from build123d import *

# Parameters (mm, degrees)
F1_DEPTH = 12
F2_DEPTH = 2.5
F3_DEPTH = 1.5


# Not quite as in the source:
# - a feature names something its author has since deleted; it is built from what else it names


with BuildPart() as f1:
    # F0 (on Top) → F1 (new body)
    with BuildSketch(Plane.XY):
        with BuildLine():
            Line((-1.9364916731, 0.5), (1.9364916731, 0.5))
            ThreePointArc((1.9364916731, 0.5), (0, 2), (-1.9364916731, 0.5))
        make_face()
        with BuildLine():
            ThreePointArc((2, 0), (1.9840593925, 0.252008585), (1.9364916731, 0.5))
            Line((1.9364916731, 0.5), (-1.9364916731, 0.5))
            ThreePointArc((-1.9364916731, 0.5), (-2, 0), (-1.9364916731, -0.5))
            Line((-1.9364916731, -0.5), (1.9364916731, -0.5))
            ThreePointArc((1.9364916731, -0.5), (1.9840593925, -0.252008585), (2, 0))
        make_face()
        with BuildLine():
            ThreePointArc((-1.9364916731, -0.5), (0, -2), (1.9364916731, -0.5))
            Line((1.9364916731, -0.5), (-1.9364916731, -0.5))
        make_face()
    extrude(amount=-F1_DEPTH)

    # F0 (on Top) → F2 (join)
    with BuildSketch(Plane.XY):
        with BuildLine():
            ThreePointArc((-3.9686269666, -0.5), (0, -4), (3.9686269666, -0.5))
            Line((3.9686269666, -0.5), (1.9364916731, -0.5))
            ThreePointArc((1.9364916731, -0.5), (0, -2), (-1.9364916731, -0.5))
            Line((-1.9364916731, -0.5), (-3.9686269666, -0.5))
        make_face()
        with BuildLine():
            Line((1.9364916731, 0.5), (3.9686269666, 0.5))
            ThreePointArc((3.9686269666, 0.5), (0, 4), (-3.9686269666, 0.5))
            Line((-3.9686269666, 0.5), (-1.9364916731, 0.5))
            ThreePointArc((-1.9364916731, 0.5), (0, 2), (1.9364916731, 0.5))
        make_face()
        with BuildLine():
            Line((-1.9364916731, 0.5), (1.9364916731, 0.5))
            ThreePointArc((1.9364916731, 0.5), (0, 2), (-1.9364916731, 0.5))
        make_face()
        with BuildLine():
            ThreePointArc((-1.9364916731, -0.5), (0, -2), (1.9364916731, -0.5))
            Line((1.9364916731, -0.5), (-1.9364916731, -0.5))
        make_face()
    extrude(amount=F2_DEPTH)

    # F0 (on Top) → F3 (join)
    with BuildSketch(Plane.XY):
        with BuildLine():
            Line((-1.9364916731, 0.5), (-3.9686269666, 0.5))
            ThreePointArc((-3.9686269666, 0.5), (-4, 0), (-3.9686269666, -0.5))
            Line((-3.9686269666, -0.5), (-1.9364916731, -0.5))
            ThreePointArc((-1.9364916731, -0.5), (-2, 0), (-1.9364916731, 0.5))
        make_face()
        with BuildLine():
            ThreePointArc((2, 0), (1.9840593925, 0.252008585), (1.9364916731, 0.5))
            Line((1.9364916731, 0.5), (-1.9364916731, 0.5))
            ThreePointArc((-1.9364916731, 0.5), (-2, 0), (-1.9364916731, -0.5))
            Line((-1.9364916731, -0.5), (1.9364916731, -0.5))
            ThreePointArc((1.9364916731, -0.5), (1.9840593925, -0.252008585), (2, 0))
        make_face()
        with BuildLine():
            ThreePointArc((3.9686269666, -0.5), (3.9921490369, -0.2504916502), (4, 0))
            ThreePointArc((4, 0), (3.9921490369, 0.2504916502), (3.9686269666, 0.5))
            Line((3.9686269666, 0.5), (1.9364916731, 0.5))
            ThreePointArc((1.9364916731, 0.5), (1.9840593925, 0.252008585), (2, 0))
            ThreePointArc((2, 0), (1.9840593925, -0.252008585), (1.9364916731, -0.5))
            Line((1.9364916731, -0.5), (3.9686269666, -0.5))
        make_face()
    extrude(amount=F3_DEPTH)


solid = f1.part
Model file for the job. Use its own axes, mm. A direction names the side the tool comes from. Coordinates: 2 decimals unless noted, no trailing zeros. Write each loop counter-clockwise with the first axis right and the second up, starting at its lowest first coordinate (ties: lowest second). Pieces come first, ordered by that corner, then holes. Notation, with made-up numbers: (-6, 26.25) - (16, 26.25) arc R31 ccw to (16, 55.25) - close; hole circle Ø4 at (62, 67). An arc over 180 degrees is marked (long way). Write each question's results on one line, items separated by ' | '. Start each with the question number.
1) Cut at B-B (z = 1). Write the cut outline in (x, y), then the cut area to 3 significant figures.
2) Probe line 1 along X through (y, z) = (-0.5, -2.25); line 2 along Z through (x, y) = (1, 3.75). List the from-to ranges inside material, lowest first. Write a range as from..to.
3) Cut at D-D (z = -10.5). Write the cut outline in (x, y).
4) Mould opens along Y. For faces 4 (the face through (0, 0.5, 2)), 5 (the face through (0, 2, 2.5)) say: pulls with the +Y half, pulls with the -Y half, needs draft (parallel to the pull), parting line crosses it, or undercut.
5) Cut at C-C (y = -1.25). Write the cut outline in (x, z), then the cut area to 3 significant figures.
6) Flat gauge pins, fed straight in: P1, Ø0.5, axis at x = 0.5, y = 0, coming from the +Z side; P2, Ø0.8, axis at x = 1, z = 2, coming from the -Y side; P3, Ø3, axis at y = -1, z = -7, coming from the +X side. Where does each tip first touch, or does it go through?
7) 3-axis set-ups, long thin cutter, end or side, ignore diameter. For faces 1 (the face through (0, -2, 2.5)), 2 (the face through (1, 2, 0)), 3 (the face through (0, -0.5, 2)): which of +Z, -Z, +X, -X, +Y, -Y reach the whole face in a straight line?
8) Cut at A-A (x = -0.5). Write the cut outline in (y, z), then the cut area to 3 significant figures.
Returned:
1) outline: circle Ø8 at (0, 0) | area: 50.3 mm^2
2) line 1: -1.94..1.94 | line 2: 0..2.5
3) outline: circle Ø4 at (0, 0)
4) face 4: undercut | face 5: needs draft
5) outline: (-3.8, 0) - (-1.56, 0) - (-1.56, -12) - (1.56, -12) - (1.56, 0) - (3.8, 0) - (3.8, 2.5) - (-3.8, 2.5) - close | area: 56.5 mm^2
6) P1: z = 1.5 | P2: y = -3.95 | P3: x = 2
7) face 1: +Z, +X, -X, +Y, -Y | face 2: -Z | face 3: +Z, +X, -X
8) outline: (-3.97, 0) - (-1.94, 0) - (-1.94, -12) - (1.94, -12) - (1.94, 0) - (3.97, 0) - (3.97, 2.5) - (0.5, 2.5) - (0.5, 1.5) - (-0.5, 1.5) - (-0.5, 2.5) - (-3.97, 2.5) - close | area: 65.3 mm^2
